For this review, use the dimensioned drawing (mm, ordinates from the lowest corner) and the shaded views. A direction names the side the tool comes from. Give positions to 0.01 mm unless a question says otherwise; leave off trailing zeros. Order: outer loops, then holes, each group sorted by start corner. A loop starts at its lowest first (then second) coordinate and runs counter-clockwise, first axis right, second up. Notation, with made-up numbers: M 83.25,-25 L 142.25,-25 A28 ccw 142.25,-3 Z; hole C 16.25,44.25 d9. An arc over 180 degrees is marked long. One line per question, with ' | ' between items. Start each with the question number.
1. The part is to be moulded in two halves that separate along Y. For the marked faces 1, 2 and 3, say which applies: +Y half, -Y half, draft (parallel to the pull), parting line (faces both ways), or undercut.
2. We need section A-A on y = 1.75. Write out the cut boundary in (x, z), then the cut area to 3 significant figures.
3. For the marked faces 4 and 5, list the 3-axis set-ups (+Z, -Z, +X, -X, +Y, -Y) from which the entire face can be reached by the end or side of a thin tool; tool diameter is ignored.
4. We need section C-C on x = 9.5. Write out the cut boundary in (y, z).
5. Insertion check: P1, Ø3, axis at y = 6.5, z = 13.5, coming from the +X side; P2, Ø3, axis at x = 16, y = 8.5, coming from the +Z side; P3, Ø2.5, axis at y = 3, z = 9, coming from the +X side; P4, Ø1.8, axis at x = 10, z = 10, coming from the -Y side. Each pin has a flat end and moves straight along its axis. Give the tip position at first contact, or say it passes through.
6. We need section B-B on z = 10. Write out the cut boundary in (x, y).
7. Wall thickness on L1, parallel to Z at x = 10, y = 11.5; L2, parallel to Y at x = 17.75, z = 5.75; L3, parallel to Z at x = 9.25, y = 12.5: over which ranges is each line inside the solid? List them lowest first.
8. We need section D-D on x = 6.5. Write out the cut boundary in (y, z).
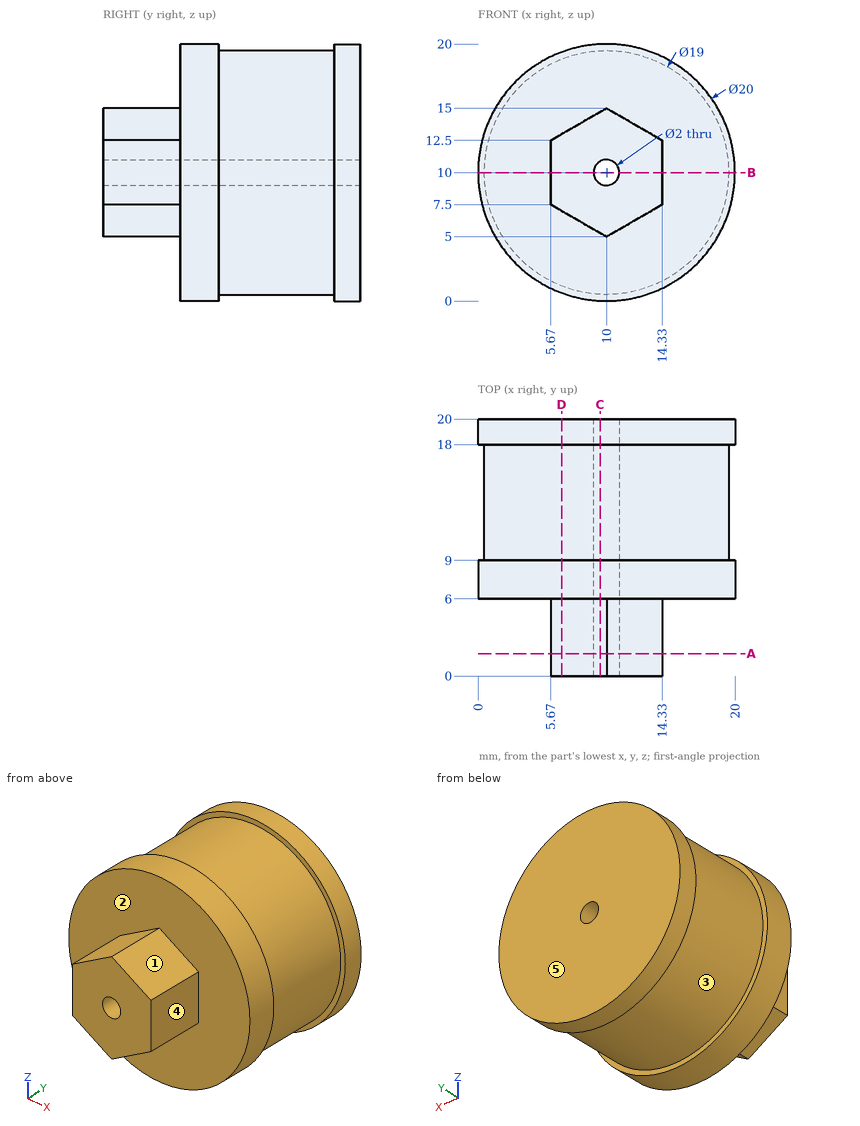
Entries:
1) face 1: draft | face 2: -Y half | face 3: undercut
2) outline: M 5.67,7.5 L 10,5 L 14.33,7.5 L 14.33,12.5 L 10,15 L 5.67,12.5 Z; hole C 10,10 d2 | area: 61.8 mm^2
3) face 4: +Z, -Z, +X, -Y | face 5: +Z, -Z, +X, -X, +Y
4) outline: M 0,5.29 L 6,5.29 L 6,0.01 L 9,0.01 L 9,0.51 L 18,0.51 L 18,0.01 L 20,0.01 L 20,9.13 L 0,9.13 Z; M 0,10.87 L 20,10.87 L 20,19.99 L 18,19.99 L 18,19.49 L 9,19.49 L 9,19.99 L 6,19.99 L 6,14.71 L 0,14.71 Z
5) P1: stops at x = 19.8 | P2: stops at z = 18.93 | P3: stops at x = 14.33 | P4: passes through
6) outline: M 0,6 L 5.67,6 L 5.67,0 L 9,0 L 9,20 L 0,20 L 0,18 L 0.5,18 L 0.5,9 L 0,9 Z; M 11,0 L 14.33,0 L 14.33,6 L 20,6 L 20,9 L 19.5,9 L 19.5,18 L 20,18 L 20,20 L 11,20 Z
7) L1: z = 0.5 to 9, 11 to 19.5 | L2: y = 6 to 20 | L3: z = 0.53 to 9.34, 10.66 to 19.47
8) outline: M 0,7.02 L 6,7.02 L 6,0.63 L 9,0.63 L 9,1.17 L 18,1.17 L 18,0.63 L 20,0.63 L 20,19.37 L 18,19.37 L 18,18.83 L 9,18.83 L 9,19.37 L 6,19.37 L 6,12.98 L 0,12.98 Z
